Here's the drawing with two shaded views (mm, measured from the low corner). I have some questions. A direction names the side the tool comes from. Give positions to 0.01 mm unless a question says otherwise; leave off trailing zeros. Loops run counter-clockwise (first coordinate to the right, second up) from the corner with the lowest first, then second, coordinate; pieces in that order, holes last. Notation, with made-up numbers: (-38, -5.75) - (-31, -5.75) arc R21 ccw to (-31, 23.25) - close; hole circle Ø10 at (44.5, -29.5). An arc over 180 degrees is marked (long way). Write each question's results on one line, items separated by ' | '. Start each with the question number.
1) If we mould it in two halves opening along Z, with no side actions, what happens to the marked faces 4, 5 and 6? For each: +Z half, -Z half, draft (parallel to the pull), parting line (faces both ways), or undercut.
2) If I drill on probe 1 along X at (y, z) = (6.7, 7.5); probe 2 along X at (y, z) = (1.55, 34); probe 3 along X at (y, z) = (2, 10), over which ranges is the centre line in solid material (lowest first)? Write a range as [from, to].
3) On a 3-axis mill with a long thin cutter (end or side, diameter ignored), from which of +Z, -Z, +X, -X, +Y, -Y can I reach the whole of each face in a straight line? I mean the marked faces 1, 2 and 3. Say none if no direction works.
4) I want a section at D-D, the plane x = 30. Write out the boundary of the cut face in (y, z), and give its area (3 significant figures).
5) I want a section at A-A, the plane z = 7.5. Write out the boundary of the cut face in (x, y), and give its area (3 significant figures).
6) I want a section at C-C, the plane y = 6.25. Write out the boundary of the cut face in (x, z), and give its area (3 significant figures).
7) I'm going to push flat-ended pins straight in: pin 1 (2.5 mm diameter, centred on x = 24, z = 34.5, fed in from +Y); pin 2 (12 mm diameter, centred on x = 37.5, z = 6, fed in from -Y); pin 3 (7 mm diameter, centred on x = 6.5, z = 7.5, fed in from -Y); pin 4 (1 mm diameter, centred on y = 8, z = 22.5, fed in from -X). Where does each tip first touch, or does it pass through?
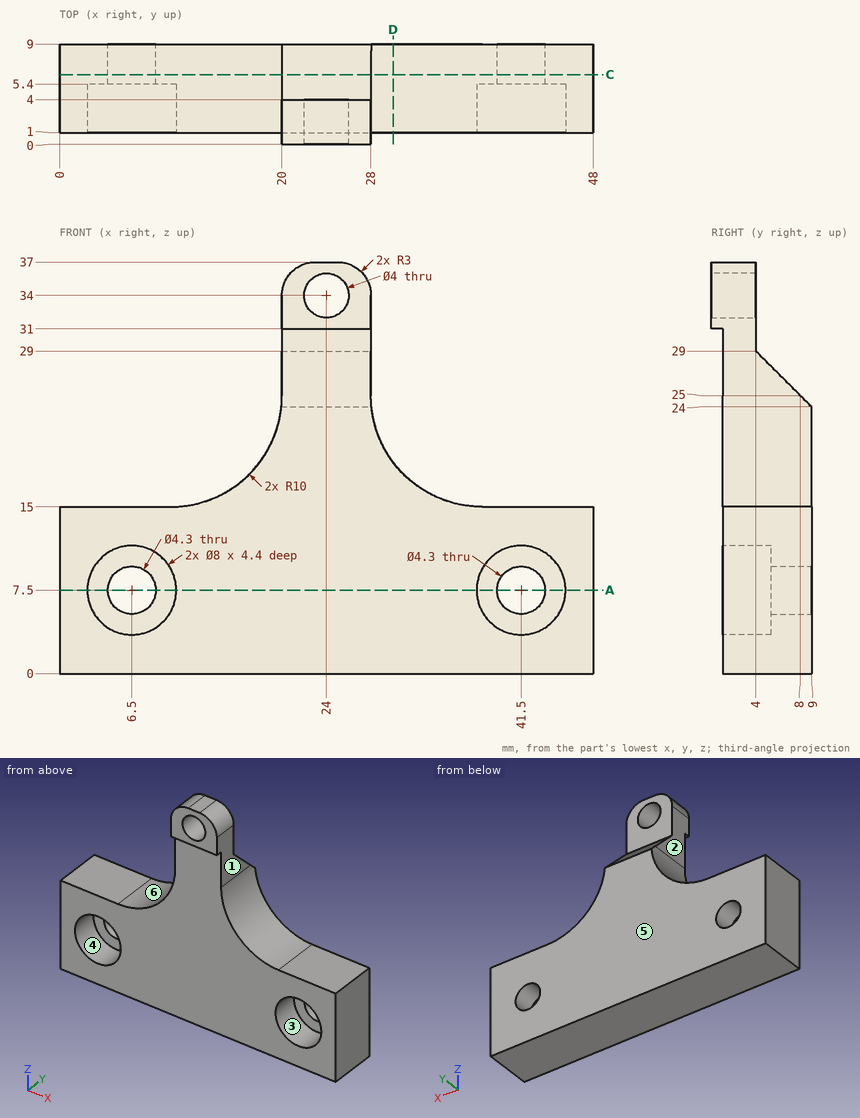
Answers:
1) face 4: undercut | face 5: draft | face 6: +Z half
2) probe 1: x = [0, 4.35], [8.65, 39.35], [43.65, 48] | probe 2: x = [20, 22], [26, 28] | probe 3: x = [0, 3.38], [9.62, 38.38], [44.62, 48]
3) face 1: +Z, +X, +Y, -Y | face 2: +Z, -X, +Y, -Y | face 3: -Y
4) outline: (1, 0) - (9, 0) - (9, 19) - (1, 19) - close | area: 152 mm2
5) outline: (0, 1) - (2.5, 1) - (2.5, 5.4) - (4.35, 5.4) - (4.35, 9) - (0, 9) - close; (8.65, 5.4) - (10.5, 5.4) - (10.5, 1) - (37.5, 1) - (37.5, 5.4) - (39.35, 5.4) - (39.35, 9) - (8.65, 9) - close; (43.65, 5.4) - (45.5, 5.4) - (45.5, 1) - (48, 1) - (48, 9) - (43.65, 9) - close | area: 283 mm2
6) outline: (0, 0) - (48, 0) - (48, 15) - (38, 15) arc R10 cw to (28, 25) - (28, 26.75) - (20, 26.75) - (20, 25) arc R10 cw to (10, 15) - (0, 15) - close; hole circle Ø4.3 at (6.5, 7.5); hole circle Ø4.3 at (41.5, 7.5) | area: 828 mm2
7) pin 1: passes through | pin 2: stops at y = 1 | pin 3: stops at y = 5.4 | pin 4: stops at x = 19.54
